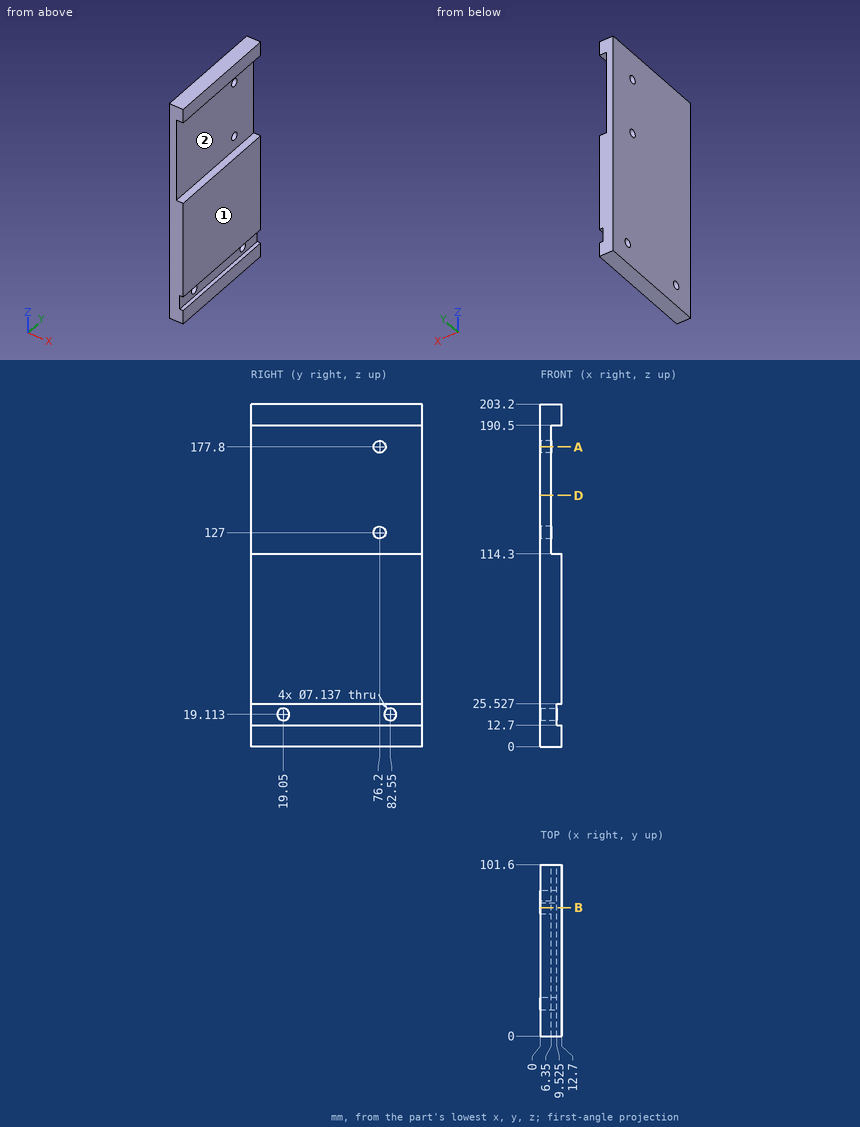
Design review of the part shown in the three views and the two pictorial views. Dimensions are in mm from the part's minimum x, y and z. Give positions to 0.01 mm unless a question says otherwise; leave off trailing zeros. Write each loop counter-clockwise with the first axis right and the second up, starting at its lowest first coordinate (ties: lowest second). Pieces come first, ordered by that corner, then holes.
(1) Mouldability with a two-part tool opening along Z and no side actions: class the marked faces 1 and 2 as +Z half, -Z half, draft (parallel to the pull), parting line (faces both ways), or undercut.
Checked values:
face 1: draft
face 2: undercut
(2) Add section B-B (y = 76.2). Give the number of separate pieces and of enclosed holes in the cut face.
Checked values:
separate pieces: 3
enclosed holes: 0
(3) Add section A-A (z = 177.8). Give the boundary of the cut face in (x, y), and give its area (3 significant figures).
Checked values:
outline: (0, 0) - (6.35, 0) - (6.35, 72.63) - (0, 72.63) - close; (0, 79.77) - (6.35, 79.77) - (6.35, 101.6) - (0, 101.6) - close
area: 600 mm2
(4) Wall thickness on line 1 along Z through (x, y) = (10.25, 39); line 2 along Z through (x, y) = (4.5, 76.2); line 3 along Y through (x, z) = (2.25, 127): over which ranges is each line inside the solid? List them lowest first.
Checked values:
line 1: z = 0 to 12.7, 25.53 to 114.3, 190.5 to 203.2
line 2: z = 0 to 123.43, 130.57 to 174.23, 181.37 to 203.2
line 3: y = 0 to 72.63, 79.77 to 101.6
(5) Clearance check with a flat-ended pin moving along its axis: pin 1 Ø9.5 at (y, z) = (82.55, 19.11) entering from +X (1 decimal). State where the tip first meets the part, or that it passes through.
Checked values:
pin 1: stops at x = 9.5
(6) Add section D-D (z = 149). Give the boundary of the cut face in (x, y).
Checked values:
outline: (0, 0) - (6.35, 0) - (6.35, 101.6) - (0, 101.6) - close
